Model file for the job. Use its own axes, mm. Face numbers are marked on the shaded views. A direction names the side the tool comes from. Round coordinates to 2 decimals unless told otherwise and drop trailing zeros. Order: outer loops, then holes, each group sorted by start corner. A loop starts at its lowest first (then second) coordinate and runs counter-clockwise, first axis right, second up. Notation, with made-up numbers: (-37, 12) - (9, 12) arc R25 ccw to (9, 50) - close; hole circle Ø7 at (7, 38). An arc over 180 degrees is marked (long way). Put each result on its own line as item: value. Start each with the question number.
Item 1: Mould opens along Y. For the marked faces 1, 2, 3 and 4 say: pulls with the +Y half, pulls with the -Y half, needs draft (parallel to the pull), parting line crosses it, or undercut.
Item 2: Pin check, flat tip, straight feed: pin 1 Ø4 at (x, z) = (12.7, 25.4) entering from +Y. Stop position of the tip, or through.
Item 3: Which spindle directions (+Z, -Z, +X, -X, +Y, -Y) get a long thin tool onto all of the face, cutting with end or side? Do the marked faces 5 and 6. Say none if no direction does.
Item 4: Saw through at C-C on y = 35.4. List the corners of the cut face in (x, z).
Item 5: Probe probe 1 along Z at (x, y) = (12.7, 1.15); probe 2 along Y at (x, z) = (0.45, 12.7); probe 3 along X at (y, z) = (10, 62). List the from-to ranges inside material, lowest first.
Item 6: Saw through at A-A on x = 22.75. List the corners of the cut face in (y, z), plus the area to 3 significant figures.
Item 7: Saw through at B-B on z = 12.7. List the corners of the cut face in (x, y), plus the area to 3 significant figures.
Item 8: Saw through at D-D on z = 50.8. List the corners of the cut face in (x, y).
Autodesk Inventor part; units mm, degrees
ref_plane "YZ Plane" through (0, 0, 0) normal (1, 0, 0) x (0, 1, 0)
ref_plane "XZ Plane" through (0, 0, 0) normal (0, 1, 0) x (-1, 0, 0)
ref_plane "XY Plane" through (0, 0, 0) normal (0, 0, 1) x (1, 0, 0)
sketch "Sketch1" plane through (0, 0, 0) normal (0, 0, 1) x (1, 0, 0)
  line L0 (0, 0) -> (25.4, 0)
  line L1 (25.4, 0) -> (25.4, 50.8)
  line L2 (25.4, 50.8) -> (0, 50.8)
  line L3 (0, 50.8) -> (0, 0)
  line L4 (1.5875, 49.2125) -> (23.8125, 49.2125)
  line L5 (23.8125, 49.2125) -> (23.8125, 1.5875)
  line L6 (23.8125, 1.5875) -> (1.5875, 1.5875)
  line L7 (1.5875, 1.5875) -> (1.5875, 49.2125)
  dimension "d0" = 25.4
  dimension "d1" = 50.8
  dimension "d2" = 1.5875
extrude "Extrusion1" add sketch "Sketch1" along normal blind 88.9
sketch "Sketch2" plane through (25.4, 0, 0) normal (1, 0, 0) x (0, 0, -1)
  line L0 (0, 0) -> (0, 50.8) construction
  line L1 (0, 50.8) -> (-12.7, 50.8) construction
  line L2 (0, 50.8) -> (-88.9, 50.8) construction
  line L3 (0, 25.4) -> (-12.7, 25.4) construction
  line L4 (-12.7, 25.4) -> (-12.7, 35.4) construction
  line L5 (-12.7, 35.4) -> (-12.7, 15.4) construction
  circle A0 centre (-12.7, 35.4) radius 3
  circle A1 centre (-12.7, 15.4) radius 3
  dimension "d5" = 12.7
  dimension "d6" = 10
  dimension "d7" = 20
  dimension "d8" = 6
extrude "Extrusion2" cut sketch "Sketch2" against normal blind 88.9
sketch "Sketch3" plane through (0, 50.8, 0) normal (0, 1, 0) x (1, 0, 0)
  line L0 (1.5875, -88.9) -> (23.8125, -88.9) construction
  line L1 (12.7, -88.9) -> (12.7, -76.2) construction
  line L2 (12.7, -76.2) -> (12.7, -50.8) construction
  line L3 (12.7, -50.8) -> (12.7, -25.4) construction
  circle A0 centre (12.7, -76.2) radius 2.5797
  circle A1 centre (12.7, -50.8) radius 2.5797
  circle A2 centre (12.7, -25.4) radius 2.5797
  point P0 (0, 0)
  dimension "d11" = 12.7
  dimension "d12" = 25.4
  dimension "d13" = 25.4
  dimension "d14" = 5.1594
extrude "Extrusion3" cut sketch "Sketch3" against normal blind 88.9
properties part number "Bumper attachment frame"
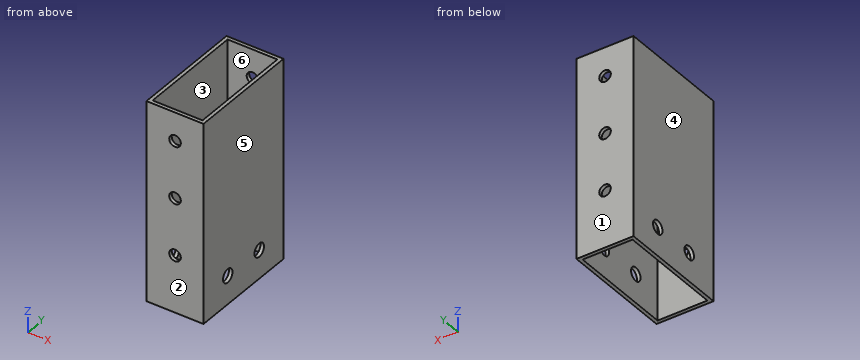
Results found:
1. face 1: pulls with the +Y half
1. face 2: pulls with the -Y half
1. face 3: undercut
1. face 4: needs draft
2. pin 1: passes through
3. face 5: +Z, -Z, +X, +Y, -Y
3. face 6: +Z, -Z
4. outline: (0, 0) - (1.59, 0) - (1.59, 9.7) - (0, 9.7) - close; (0, 15.7) - (1.59, 15.7) - (1.59, 88.9) - (0, 88.9) - close; (23.81, 0) - (25.4, 0) - (25.4, 9.7) - (23.81, 9.7) - close; (23.81, 15.7) - (25.4, 15.7) - (25.4, 88.9) - (23.81, 88.9) - close
5. probe 1: z = 0 to 22.82, 27.98 to 48.22, 53.38 to 73.62, 78.78 to 88.9
5. probe 2: y = 0 to 12.4, 18.4 to 32.4, 38.4 to 50.8
5. probe 3: x = 0 to 1.59, 23.81 to 25.4
6. outline: (0, 0) - (1.59, 0) - (1.59, 88.9) - (0, 88.9) - close; (49.21, 0) - (50.8, 0) - (50.8, 88.9) - (49.21, 88.9) - close
6. area: 282 mm²
7. outline: (0, 0) - (25.4, 0) - (25.4, 12.4) - (23.81, 12.4) - (23.81, 1.59) - (1.59, 1.59) - (1.59, 12.4) - (0, 12.4) - close; (0, 18.4) - (1.59, 18.4) - (1.59, 32.4) - (0, 32.4) - close; (0, 38.4) - (1.59, 38.4) - (1.59, 49.21) - (23.81, 49.21) - (23.81, 38.4) - (25.4, 38.4) - (25.4, 50.8) - (0, 50.8) - close; (23.81, 18.4) - (25.4, 18.4) - (25.4, 32.4) - (23.81, 32.4) - close
7. area: 194 mm²
8. outline: (0, 0) - (10.12, 0) - (10.12, 1.59) - (1.59, 1.59) - (1.59, 49.21) - (10.12, 49.21) - (10.12, 50.8) - (0, 50.8) - close; (15.28, 0) - (25.4, 0) - (25.4, 50.8) - (15.28, 50.8) - (15.28, 49.21) - (23.81, 49.21) - (23.81, 1.59) - (15.28, 1.59) - close
